Study the drawing (mm; zero at the part's minimum x, y, z) and answer. A direction names the side the tool comes from. Round coordinates to 2 decimals unless told otherwise and drop trailing zeros. Order: outer loops, then holes, each group sorted by start corner. A loop starts at its lowest first (then second) coordinate and runs counter-clockwise, first axis right, second up. Notation, with made-up numbers: (-0.5, 36) - (3.5, 36) arc R23 ccw to (3.5, 48) - close; hole circle Ø5 at (-39.5, 49.25). An arc over 180 degrees is marked (long way). Put each result on its own line as item: value. Start each with the question number.
Q1. Section C-C on x = 127 is taken. Give the vertices of the cut face in (y, z), then the cut area to 3 significant figures.
Q2. Section A-A on y = 40 is taken. Give the vertices of the cut face in (x, z) (3 decimals), then the cut area to 3 significant figures.
Q3. Each of these flat-tipped pins is pushed along its axis until it touches: pin 1 Ø12 at (y, z) = (85, 153) entering from -X; pin 2 Ø2 at (x, z) = (143.5, 117) entering from -Y; pin 3 Ø9.5 at (x, z) = (130, 80) entering from -Y. Where does it stop, or does it pass through?
Q4. Find the intervals of material crossed by line 1 along Z through (x, y) = (127, 115); line 2 along Z through (x, y) = (108, 116); line 3 along X through (y, z) = (58, 203), in increasing order. Write a range as from..to.
Q5. For a pull along Z with two mould halves and no side action, classify the marked faces 1, 2 and 3 as pulls with the +Z half, pulls with the -Z half, needs draft (parallel to the pull), parting line crosses it, or undercut.
Q6. Section D-D on z = 194 is taken. Give the vertices of the cut face in (x, y), then the cut area to 3 significant figures.
Q7. Which of the six approach directions +Z, -Z, +X, -X, +Y, -Y give full straight-line access (tool end or side, diameter ignored) to the marked faces 4, 5 and 6?
Q8. Section B-B on y = 142 is taken. Give the vertices of the cut face in (x, z).
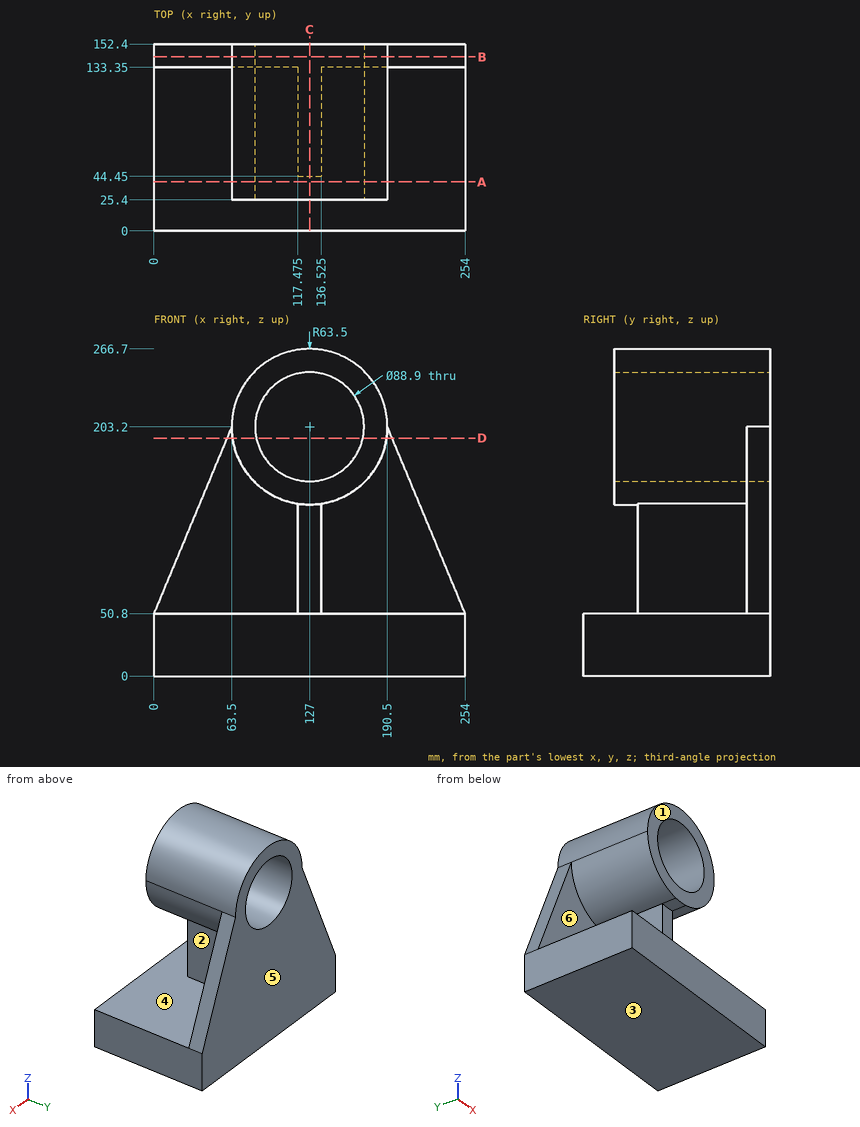
Findings:
1. outline: (0, 0) - (152.4, 0) - (152.4, 158.75) - (25.4, 158.75) - (25.4, 139.7) - (44.45, 139.7) - (44.45, 50.8) - (0, 50.8) - close; (25.4, 247.65) - (152.4, 247.65) - (152.4, 266.7) - (25.4, 266.7) - close
1. area: 22,200 mm2
2. outline: (0, 0) - (254, 0) - (254, 50.8) - (0, 50.8) - close; (63.5, 203.2) arc R63.5 ccw to (117.475, 140.418) arc R63.5 ccw to (136.525, 140.418) arc R63.5 ccw to (190.5, 203.2) arc R63.5 ccw to start; hole circle Ø88.9 at (127, 203.2)
2. area: 19,400 mm2
3. pin 1: x = 81.41
3. pin 2: y = 133.35
3. pin 3: y = 44.45
4. line 1: 0..158.75, 247.65..266.7
4. line 2: 0..50.8, 142.61..163.02, 243.38..263.79
4. line 3: 63.5..82.55, 171.45..190.5
5. face 1: needs draft
5. face 2: undercut
5. face 3: pulls with the -Z half
6. outline: (59.67, 133.35) - (64.17, 133.35) - (64.17, 25.4) - (83.51, 25.4) - (83.51, 152.4) - (59.67, 152.4) - close; (170.49, 25.4) - (189.83, 25.4) - (189.83, 133.35) - (194.33, 133.35) - (194.33, 152.4) - (170.49, 152.4) - close
6. area: 5,080 mm2
7. face 4: -Y
7. face 5: +Z, -Z, +X, -X, +Y
7. face 6: -X, -Y
8. outline: (0, 0) - (254, 0) - (254, 50.8) - (190.5, 203.2) arc R63.5 ccw to (63.5, 203.2) - (0, 50.8) - close; hole circle Ø88.9 at (127, 203.2)
